from build123d import *

# Parameters (mm, degrees)
F1_DEPTH = 13
F3_D     = 3.2
F4_T     = -2.8
F6_DEPTH = 40.001
F7_DEPTH = 2.5
F8_R     = 3


with BuildPart() as f1:
    # F0 (on Right) → F1 (new body)
    with BuildSketch(Plane.YZ):
        with BuildLine():
            ThreePointArc((-17, 72), (-19.1213203436, 71.1213203436), (-20, 69))
            Line((-20, 69), (-20, 25))
            ThreePointArc((-20, 25), (-19.8196101249, 17.5795865345), (-19.2788666706, 10.1767037836))
            Line((-19.2788666706, 10.1767037836), (-18.1140558503, -1.7666297441))
            ThreePointArc((-18.1140558503, -1.7666297441), (-13.8130173627, -11.8507616353), (-4.5, -17.6349085623))
            Line((-4.5, -17.6349085623), (-4.5, -26.6349085623))
            Line((-4.5, -26.6349085623), (-0.5, -26.6349085623))
            Line((-0.5, -26.6349085623), (-0.5, -14.1911944529))
            ThreePointArc((-0.5, -14.1911944529), (-14.1977984426, 0.2500387658), (0, 14.2))
            ThreePointArc((0, 14.2), (14.1977984426, 0.2500387658), (0.5, -14.1911944529))
            Line((0.5, -14.1911944529), (0.5, -26.6349085623))
            Line((0.5, -26.6349085623), (4.5, -26.6349085623))
            Line((4.5, -26.6349085623), (4.5, -17.6349085623))
            ThreePointArc((4.5, -17.6349085623), (13.8130173627, -11.8507616353), (18.1140558503, -1.7666297441))
            Line((18.1140558503, -1.7666297441), (19.2788666706, 10.1767037836))
            Line((19.2788666706, 10.1767037836), (20, 25))
            Line((20, 25), (20, 69))
            ThreePointArc((20, 69), (19.1213203436, 71.1213203436), (17, 72))
            Line((17, 72), (0, 72))
            Line((0, 72), (-17, 72))
        make_face()
        with BuildLine():
            Line((-17.2, 26.5), (-17.2, 36.5))
            ThreePointArc((-17.2, 36.5), (-15.5, 38.2), (-13.8, 36.5))
            Line((-13.8, 36.5), (-13.8, 26.5))
            ThreePointArc((-13.8, 26.5), (-15.5, 24.8), (-17.2, 26.5))
        make_face(mode=Mode.SUBTRACT)
        with BuildLine():
            Line((-17.2, 57.5), (-17.2, 67.5))
            ThreePointArc((-17.2, 67.5), (-15.5, 69.2), (-13.8, 67.5))
            Line((-13.8, 67.5), (-13.8, 57.5))
            ThreePointArc((-13.8, 57.5), (-15.5, 55.8), (-17.2, 57.5))
        make_face(mode=Mode.SUBTRACT)
        with BuildLine():
            ThreePointArc((-11.25, 52), (-7.9549512883, 59.9549512883), (0, 63.25))
            ThreePointArc((0, 63.25), (7.9549512883, 59.9549512883), (11.25, 52))
            Line((11.25, 52), (11.25, 42))
            ThreePointArc((11.25, 42), (7.9549512883, 34.0450487117), (0, 30.75))
            ThreePointArc((0, 30.75), (-7.9549512883, 34.0450487117), (-11.25, 42))
            Line((-11.25, 42), (-11.25, 52))
        make_face(mode=Mode.SUBTRACT)
        with BuildLine():
            ThreePointArc((17.2, 26.5), (15.5, 24.8), (13.8, 26.5))
            Line((13.8, 26.5), (13.8, 36.5))
            ThreePointArc((13.8, 36.5), (15.5, 38.2), (17.2, 36.5))
            Line((17.2, 36.5), (17.2, 26.5))
        make_face(mode=Mode.SUBTRACT)
        with BuildLine():
            Line((17.2, 67.5), (17.2, 57.5))
            ThreePointArc((17.2, 57.5), (15.5, 55.8), (13.8, 57.5))
            Line((13.8, 57.5), (13.8, 67.5))
            ThreePointArc((13.8, 67.5), (15.5, 69.2), (17.2, 67.5))
        make_face(mode=Mode.SUBTRACT)
    extrude(amount=F1_DEPTH)

    # F3 (through all)
    with Locations(Plane.XZ.offset(4.5)):
        with Locations((4.5, -22.1349085623)):
            Hole(F3_D / 2)

    # F4
    f4_openings = [f1.faces().sort_by_distance(p)[0] for p in [
        (13, -0.017595, 30.158795),
    ]]
    offset(amount=F4_T, openings=f4_openings)

    # F5 (on face) → F6 (cut, through all)
    with BuildSketch(Plane.XZ.offset(20)):
        Polygon((13, -28), (13, 22), (9, 18.6436014753), (9, -28), align=None)
    extrude(amount=-F6_DEPTH, mode=Mode.SUBTRACT)

    # F2 (on face) → F7 (cut)
    with BuildSketch(Plane.XZ.offset(4.5)):
        Polygon((6.1454482672, -19.2849085623), (2.8545517328, -19.2849085623), (1.2091034656, -22.1349085623), (4.5, -22.1349085623), (4.5, -24.9849085623), (6.1454482672, -24.9849085623), (7.7908965344, -22.1349085623), align=None)
        Polygon((4.5, -22.1349085623), (1.2091034656, -22.1349085623), (2.8545517328, -24.9849085623), (4.5, -24.9849085623), align=None)
    extrude(amount=-F7_DEPTH, mode=Mode.SUBTRACT)

    # F8
    f8_edges = [f1.edges().sort_by_distance(p)[0] for p in [
        (0, -2.5, -26.634909),
        (0, 2.5, -26.634909),
        (9, -2.5, -26.634909),
        (9, 2.5, -26.634909),
    ]]
    fillet(f8_edges, radius=F8_R)


solid = f1.part
The model under review builds one solid part; all positions refer to its coordinate system, in mm. A direction names the side the tool comes from. Coordinates: 2 decimals unless noted, no trailing zeros. Loops run counter-clockwise (first coordinate to the right, second up) from the corner with the lowest first, then second, coordinate; pieces in that order, holes last. Notation, with made-up numbers: (29.5, -9) -> (40.5, -9) arc R11 cw to (40.5, 6) -> close; hole circle Ø6 at (36.25, 56.5). An arc over 180 degrees is marked (long way). Use a Markdown table: item, result. Add a question column.
1. Add section C-C on y = 8.5. Write out the cut boundary in (x, z), plus the area to 3 significant figures.
2. Machinability: for faces 1 (the face through (8, 0, 69.2)), 2 (the face through (6, -17.2, 62)), 3 (the face through (4, 4.5, -20)), 4 (the face through (6.957, -3.268, -23.58)), which of the approach directions +Z, -Z, +X, -X, +Y, -Y give a long, thin tool a straight path to every point of the face, cutting with its end or side? Answer none if there is none.
3. Add section B-B on z = -7.5. Write out the cut boundary in (x, y).
4. Add section A-A on y = 3.5. Write out the cut boundary in (x, z), plus the area to 3 significant figures.
5. Draft analysis for pull direction Y (two halves, no side actions). For faces 5 (the face through (0.855, 2.528, -25.733)), 6 (the face through (4, 0.5, -20)), 7 (the face through (6, -20, 47)), state which applies: pulls with the +Y half, pulls with the -Y half, needs draft (parallel to the pull), parting line crosses it, or undercut.
6. Clearance check with flat-ended pins moving along their axes: pin 1 Ø10 at (y, z) = (-15, 3.5) entering from +X; pin 2 Ø3 at (x, z) = (4.5, -23) entering from -Y; pin 3 Ø2 at (x, z) = (9, 22) entering from +Y; pin 4 Ø5 at (y, z) = (0, 10) entering from -X. State where each tip first meets the part, or that it passes through.
7. Add section D-D on x = 4.5. Give the number of separate pieces and of enclosed holes in the cut face, plus the area to 3 significant figures.
8. To check wall thickness, follow line 1 (Y direction, x = 1.75, z = 67); line 2 (Y direction, x = 5.75, z = 46.5); line 3 (Y direction, x = 2.5, z = 51.5). State the ranges of each line that lie inside material, in increasing order.
Returned:
| question | item | result |
|---|---|---|
| 1 | outline | (0, -16.09) -> (9, -16.09) -> (9, -11.37) -> (0, -11.37) -> close; (0, 11.37) -> (9, 11.37) -> (9, 14.72) -> (2.8, 14.72) -> (2.8, 30.81) -> (13, 30.81) -> (13, 34.63) -> (0, 34.63) -> close; (0, 59.37) -> (13, 59.37) -> (13, 63.19) -> (2.8, 63.19) -> (2.8, 69.2) -> (13, 69.2) -> (13, 72) -> (0, 72) -> close |
| 1 | area | 270 mm² |
| 2 | face 1 | +X |
| 2 | face 2 | +X, -X |
| 2 | face 3 | -Z, +X, -X, +Y |
| 2 | face 4 | -Y |
| 3 | outline | (0, -16.58) -> (9, -16.58) -> (9, -12.06) -> (0, -12.06) -> close; (0, 12.06) -> (9, 12.06) -> (9, 16.58) -> (0, 16.58) -> close |
| 4 | outline | (0, -23.63) arc R3 ccw to (3, -26.63) -> (6, -26.63) arc R3 ccw to (9, -23.63) -> (9, -13.76) -> (0, -13.76) -> close; (0, 13.76) -> (9, 13.76) -> (9, 16.64) -> (2.8, 16.64) -> (2.8, 28.39) -> (13, 28.39) -> (13, 31.31) -> (0, 31.31) -> close; (0, 62.69) -> (13, 62.69) -> (13, 65.61) -> (2.8, 65.61) -> (2.8, 69.2) -> (13, 69.2) -> (13, 72) -> (0, 72) -> close; hole circle Ø3.2 at (4.5, -22.13) |
| 4 | area | 285 mm² |
| 5 | face 5 | needs draft |
| 5 | face 6 | undercut |
| 5 | face 7 | pulls with the -Y half |
| 6 | pin 1 | stops at x = 9 |
| 6 | pin 2 | stops at y = -2 |
| 6 | pin 3 | stops at y = 19.9 |
| 6 | pin 4 | passes through |
| 7 | separate pieces | 3 |
| 7 | enclosed holes | 9 |
| 7 | area | 1,330 mm² |
| 8 | line 1 | y = -20 to -17.2, -13.8 to 13.8, 17.2 to 20 |
| 8 | line 2 | y = -20 to -17.2, -14.05 to -11.25, 11.25 to 14.05, 17.2 to 20 |
| 8 | line 3 | y = -20 to -11.25, 11.25 to 20 |
